from build123d import *

# Parameters (mm, degrees)
ESBO_O1_W                = 38
ESBO_O1_H                = 12
ESBO_O1_R                = 2
RESSALTO_EXTRUS_O1_DEPTH = 1.5


with BuildPart() as part:
    # Esboço1 → Ressalto-extrusão1 (new body)
    with BuildSketch(Plane(origin=(0, 0, 0), x_dir=(0, 0, -1), z_dir=(1, 0, 0))):
        Rectangle(ESBO_O1_W, ESBO_O1_H)
        with Locations((-14, 0)):
            Circle(ESBO_O1_R, mode=Mode.SUBTRACT)
        with Locations(Location((14, 0, 0), (0, 0, 180))):
            Circle(ESBO_O1_R, mode=Mode.SUBTRACT)
    extrude(amount=RESSALTO_EXTRUS_O1_DEPTH)


solid = part.part
CAD build for the part. Positions are in the model's coordinates, mm. Round coordinates to 2 decimals unless told otherwise and drop trailing zeros. Loops run counter-clockwise (first coordinate to the right, second up) from the corner with the lowest first, then second, coordinate; pieces in that order, holes last.
(1) Cut at B-B (z = -14). Give the cut face in (x, y), plus the area to 3 significant figures.
(2) Cut at C-C (x = 1.2). Give the cut face in (y, z), plus the area to 3 significant figures.
(3) Drop a flat-ended pin along its axis: pin 1 (6.5 mm diameter, centred on y = 0, z = 14, fed in from -X). Give the stop position or say it passes through.
(4) Wall check: line 1 along Y through (x, z) = (0.65, -14); line 2 along Z through (x, y) = (0.6, -1.75); line 3 along Y through (x, z) = (0.2, 13). Give the ranges that are in metal, low to high.
(5) Two-plate mould, pull along Y, no slides. Class faces 1 (the flat face through (1, 0, -19)), 2 (the flat face through (1, 6, 0)), 3 (the cylindrical face through (0.7, -1.2, 15.6)): +Y half, -Y half, draft (parallel to the pull), parting line (faces both ways), or undercut.
(6) Cut at A-A (y = 0). Give the cut face in (x, z), plus the area to 3 significant figures.
Findings below:
1. outline: (0, -6) - (1.5, -6) - (1.5, -2) - (0, -2) - close; (0, 2) - (1.5, 2) - (1.5, 6) - (0, 6) - close
1. area: 12.0 mm2
2. outline: (-6, -19) - (6, -19) - (6, 19) - (-6, 19) - close; hole circle Ø4 at (0, -14); hole circle Ø4 at (0, 14)
2. area: 431 mm2
3. pin 1: stops at x = 0
4. line 1: y = -6 to -2, 2 to 6
4. line 2: z = -19 to -14.97, -13.03 to 13.03, 14.97 to 19
4. line 3: y = -6 to -1.73, 1.73 to 6
5. face 1: draft
5. face 2: +Y half
5. face 3: undercut
6. outline: (0, -19) - (1.5, -19) - (1.5, -16) - (0, -16) - close; (0, -12) - (1.5, -12) - (1.5, 12) - (0, 12) - close; (0, 16) - (1.5, 16) - (1.5, 19) - (0, 19) - close
6. area: 45.0 mm2
